Part print with two shaded views. Sizes in mm from the minimum x, y, z corner. A direction names the side the tool comes from. Round coordinates to 2 decimals unless told otherwise and drop trailing zeros. Write each loop counter-clockwise with the first axis right and the second up, starting at its lowest first coordinate (ties: lowest second). Pieces come first, ordered by that corner, then holes. Notation, with made-up numbers: (-7, -26.75) -> (36, -26.75) arc R19 ccw to (36, -3.75) -> close; hole circle Ø2 at (5.5, 30.25). An arc over 180 degrees is marked (long way). Return JSON: item names as keys, results as strings.
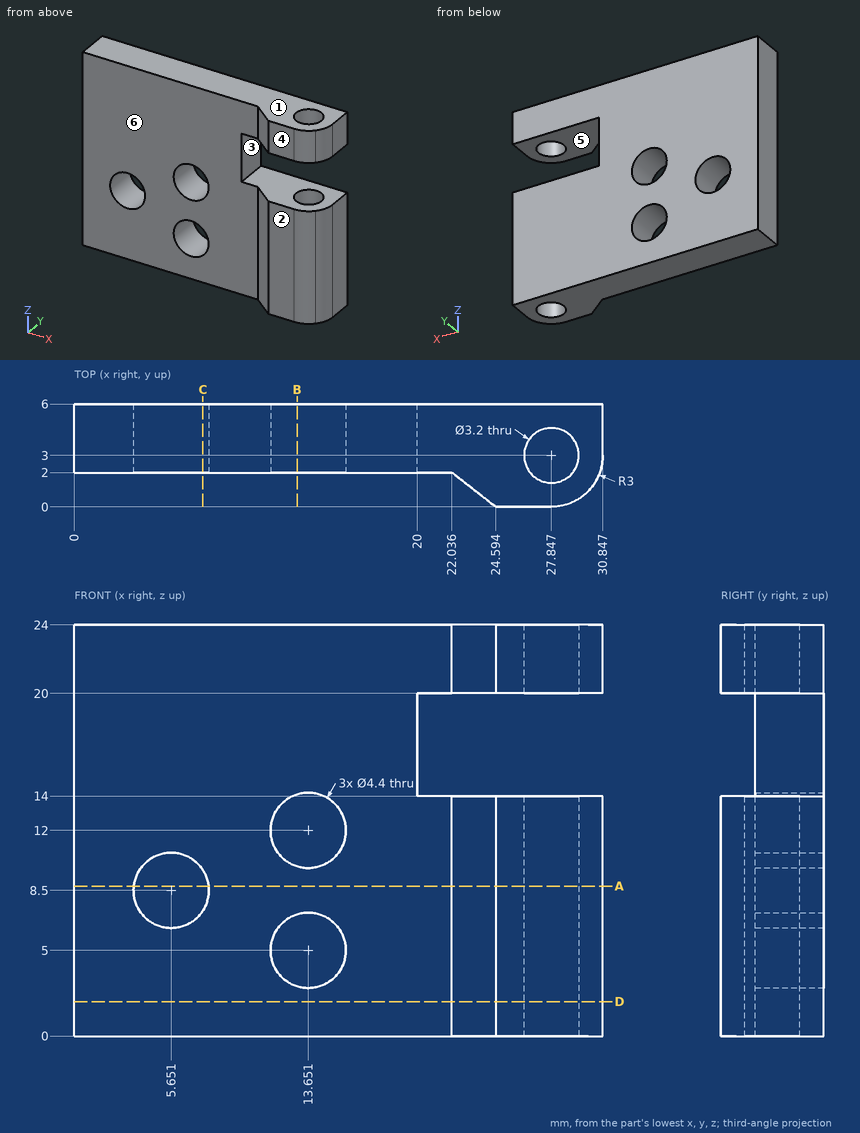
Q1. Wall check: L1, parallel to Z at x = 13.5, y = 3.55 (1 decimal); L2, parallel to Z at x = 25, y = 0.35; L3, parallel to X at y = 2.85, z = 2 (1 decimal). Give the ranges that are in metal, low to high.
Verdict:
{"L1": "z = 0 to 2.8, 7.2 to 9.8, 14.2 to 24", "L2": "z = 0 to 14, 20 to 24", "L3": "x = 0 to 26.3, 29.4 to 30.8"}
Q2. Saw through at C-C on x = 7.5. List the corners of the cut face in (y, z).
Verdict:
{"outline": "(2, 0) -> (6, 0) -> (6, 7.31) -> (2, 7.31) -> close; (2, 9.69) -> (6, 9.69) -> (6, 24) -> (2, 24) -> close"}
Q3. Two-plate mould, pull along Z, no slides. Class the marked faces 1, 2 and 3: +Z half, -Z half, draft (parallel to the pull), parting line (faces both ways), or undercut.
Verdict:
{"face 1": "+Z half", "face 2": "draft", "face 3": "undercut"}
Q4. Pin check, flat tips, straight feed: pin 1 Ø5 at (x, z) = (7.5, 19.5) entering from -Y; pin 2 Ø5 at (x, z) = (24.5, 15) entering from -Y. Stop position of each tip, or through.
Verdict:
{"pin 1": "stops at y = 2", "pin 2": "stops at y = 0"}
Q5. 3-axis set-ups, long thin cutter, end or side, ignore diameter. For the marked faces 4, 5 and 6: which of +Z, -Z, +X, -X, +Y, -Y reach the whole face in a straight line?
Verdict:
{"face 4": "+Z, -Z, +X, -X, -Y", "face 5": "+X, +Y, -Y", "face 6": "+Z, -Z, -X, -Y"}
Q6. Saw through at B-B on x = 13. List the corners of the cut face in (y, z).
Verdict:
{"outline": "(2, 0) -> (6, 0) -> (6, 2.9) -> (2, 2.9) -> close; (2, 7.1) -> (6, 7.1) -> (6, 9.9) -> (2, 9.9) -> close; (2, 14.1) -> (6, 14.1) -> (6, 24) -> (2, 24) -> close"}
Q7. Saw through at D-D on z = 2. List the corners of the cut face in (x, y) (1 decimal).
Verdict:
{"outline": "(0, 2) -> (22, 2) -> (24.6, 0) -> (27.8, 0) arc R3 ccw to (30.8, 3) -> (30.8, 6) -> (0, 6) -> close; hole circle Ø3.2 at (27.8, 3)"}
Q8. Saw through at A-A on z = 8.75. List the corners of the cut face in (x, y) (1 decimal).
Verdict:
{"outline": "(0, 2) -> (3.5, 2) -> (3.5, 6) -> (0, 6) -> close; (7.8, 2) -> (22, 2) -> (24.6, 0) -> (27.8, 0) arc R3 ccw to (30.8, 3) -> (30.8, 6) -> (7.8, 6) -> close; hole circle Ø3.2 at (27.8, 3)"}
